Check sheet for the modelled part. Datum: model origin and axes. Units: mm. Round coordinates to 2 decimals unless told otherwise and drop trailing zeros. Loops run counter-clockwise (first coordinate to the right, second up) from the corner with the lowest first, then second, coordinate; pieces in that order, holes last. Notation, with made-up numbers: (-17.75, 28.25) -> (-7.75, 28.25) arc R24 cw to (-7.75, 51.25) -> close; hole circle Ø6 at (66, -34). An arc over 180 degrees is marked (long way). Use one line per item in the form item = value. Start each with the question number.
(1) Go/stop test with flat-tipped pins: pin 1 (1 mm diameter, centred on y = 2, z = -2, fed in from -X); pin 2 (3 mm diameter, centred on x = 3, z = 7, fed in from -Y). Record where each tip stops, or that it passes through.
(2) Sectioned sample at D-D (z = 0). Record the cut outline in (x, y), and give its area (3 significant figures).
(3) Sectioned sample at C-C (y = 1.5). Record the cut outline in (x, z).
(4) Sectioned sample at A-A (x = 0). Record the cut outline in (y, z), and give its area (3 significant figures).
(5) Material ranges on probe 1 along Z at (x, y) = (0, 1.75); probe 2 along X at (y, z) = (0.8, -10); probe 3 along Z at (x, y) = (1, 1.95), recorded low to high. Write a range as [from, to].
(6) Sectioned sample at B-B (z = 10). Record the cut outline in (x, y).
(7) Draft check along X on faces 1 (the flat face through (0, 3, -6)), 2 (the conical face through (9.2, 2.8, -0.2)), 3 (the cylindrical face through (0.16, 1.48, -11.24)). Enter one of: released by +X, released by -X, zero draft, split by the parting line, or undercut.
Autodesk Inventor part; units mm, degrees
ref_plane "YZ Plane" through (0, 0, 0) normal (1, 0, 0) x (0, 1, 0)
ref_plane "XZ Plane" through (0, 0, 0) normal (0, 1, 0) x (-1, 0, 0)
ref_plane "XY Plane" through (0, 0, 0) normal (0, 0, 1) x (1, 0, 0)
sketch "스케치1" plane through (0, 0, 0) normal (0, 1, 0) x (-1, 0, 0)
  circle A0 centre (0, 0) radius 10
  circle A1 centre (0, 10) radius 1.25
  circle A2 centre (0, 10) radius 3
  line L0 (0, 0) -> (3.5124, 0)
  circle A3 centre (0, -10) radius 1.25
  circle A4 centre (0, -10) radius 3
  circle A5 centre (0, 0) radius 5.5
  point P0 (2.9661, 9.55)
  point P1 (-2.9661, 9.55)
  point P2 (-2.9661, -9.55)
  point P3 (2.9661, -9.55)
  dimension "d0" = 20
  dimension "d2" = 2.5
  dimension "d3" = 6
  dimension "d4" = 11
extrude "돌출1" add sketch "스케치1" along normal blind 3 contours A0 A4 A2 | A2 A0 A1 | A0 A1 A2 | A4 A0 A3 | A0 A3 A4
chamfer "모따기1" distance 1 angle 45 2 edges at (10, 3, 0) (-10, 3, 0)
properties part number "책상 고정판 홀더"
Checks:
q1.pin_1 = -9.89
q1.pin_2 = 0
q2.outline = (-10, 0) -> (-5.5, 0) -> (-5.5, 3) -> (-9, 3) -> (-10, 2) -> close; (5.5, 0) -> (10, 0) -> (10, 2) -> (9, 3) -> (5.5, 3) -> close
q2.area = 26.0 mm2
q3.outline = (-2.97, -9.55) arc R3 ccw (long way) to (2.97, -9.55) arc R10 ccw to (2.97, 9.55) arc R3 ccw (long way) to (-2.97, 9.55) arc R10 ccw to start; hole circle Ø11 at (0, 0); hole circle Ø2.5 at (0, -10); hole circle Ø2.5 at (0, 10)
q4.outline = (0, -13) -> (3, -13) -> (3, -11.25) -> (0, -11.25) -> close; (0, -8.75) -> (3, -8.75) -> (3, -5.5) -> (0, -5.5) -> close; (0, 5.5) -> (3, 5.5) -> (3, 8.75) -> (0, 8.75) -> close; (0, 11.25) -> (3, 11.25) -> (3, 13) -> (0, 13) -> close
q4.area = 30.0 mm2
q5.probe_1 = [-13, -11.25], [-8.75, -5.5], [5.5, 8.75], [11.25, 13]
q5.probe_2 = [-3, -1.25], [1.25, 3]
q5.probe_3 = [-12.83, -10.75], [-9.25, -5.41], [5.41, 9.25], [10.75, 12.83]
q6.outline = (-3, 0) -> (-1.25, 0) -> (-1.25, 3) -> (-3, 3) -> close; (1.25, 0) -> (3, 0) -> (3, 3) -> (1.25, 3) -> close
q7.face_1 = zero draft
q7.face_2 = released by +X
q7.face_3 = undercut
